Input: part model. Units: mm. Frame: model coordinates. A direction names the side the tool comes from. Coordinates: 2 decimals unless noted, no trailing zeros. Loops run counter-clockwise (first coordinate to the right, second up) from the corner with the lowest first, then second, coordinate; pieces in that order, holes last. Notation, with made-up numbers: (52.5, 26) -> (108.5, 26) arc R24 cw to (108.5, 59) -> close; hole circle Ø8 at (3, 87.25). An arc over 180 degrees is marked (long way). Answer as a JSON object with one key per item and string values.
from build123d import *

# Parameters (mm, degrees)
CROQUIS1_R              = 5.05
CROQUIS1_R_2            = 1.7500000000000002
SALIENTE_EXTRUIR1_DEPTH = 1.5
CROQUIS8_R              = 7
CROQUIS8_R_2            = 3.5499999999999994
SALIENTE_EXTRUIR5_DEPTH = 1.5
CROQUIS9_R              = 3
CORTAR_EXTRUIR3_DEPTH   = 1.5
CROQUIS10_R             = 3.55
SALIENTE_EXTRUIR6_DEPTH = 0.4
CHAFL_N1_SIZE           = 0.5


with BuildPart() as part:
    # Croquis1 → Saliente-Extruir1 (new body)
    with BuildSketch(Plane.XY):
        with BuildLine():
            Line((3.75, -2.0000000000000004), (19.8, -2))
            Line((19.8, -2), (19.8, 2))
            Line((19.8, 2), (8.90555127546391, 2))
            ThreePointArc((8.905551275463925, 1.9999999999999556), (6.887272990754048, 14.817665616090519), (-0.5849400470518447, 4.209554031171866))
            ThreePointArc((-0.5849400470518499, 4.209554031171828), (-3.484830188538549, -2.4327882269220193), (3.7499999999999996, -2.0000000000000013))
        make_face()
        with Locations((5.299999999999999, 8)):
            Circle(CROQUIS1_R, mode=Mode.SUBTRACT)
        Circle(CROQUIS1_R_2, mode=Mode.SUBTRACT)
    extrude(amount=SALIENTE_EXTRUIR1_DEPTH)

    # Croquis8 → Saliente-Extruir5 (add)
    with BuildSketch(Plane.XY.offset(1.5)):
        with Locations(Location((5.299999999999999, 8, 0), (0, 0, 212.785282787))):
            Circle(CROQUIS8_R)
        with Locations((5.299999999999999, 8)):
            Circle(CROQUIS8_R_2, mode=Mode.SUBTRACT)
    extrude(amount=SALIENTE_EXTRUIR5_DEPTH)

    # Croquis9 → Cortar-Extruir3 (cut)
    with BuildSketch(Plane.XY.offset(1.5)):
        Circle(CROQUIS9_R)
    extrude(amount=CORTAR_EXTRUIR3_DEPTH, mode=Mode.SUBTRACT)

    # Croquis10 → Saliente-Extruir6 (add)
    with BuildSketch(Plane(origin=(0, 0, 1.5), x_dir=(-1, 0, 0), z_dir=(0, 0, -1))):
        with Locations((-5.299999999999999, 8)):
            Circle(CROQUIS10_R)
    extrude(amount=-SALIENTE_EXTRUIR6_DEPTH)

    # Simetría1: part across plane


with BuildPart() as part_1:
    add(part.part)
    add(part.part.mirror(Plane(origin=(19.8, 0, 1.5), x_dir=(0, 0, 1), z_dir=(1, 0, 0))))

    # Chaflán1
    chafl_n1_edges = [part_1.edges().sort_by_distance(p)[0] for p in [
        (19.8, -2.000000000000001, 0),
        (-3.484830188538548, -2.4327882269220202, 0),
        (6.887272990754054, 14.817665616090517, 0),
        (41.35, 2.1e-16, 0),
        (39.35, 8, 0),
        (32.712727009245945, 14.817665616090517, 0),
        (43.08483018853855, -2.4327882269220202, 0),
        (0.2499999999999991, 8, 0),
        (-1.7500000000000002, 2.1e-16, 0),
        (19.8, 1.999999999999977, 0),
    ]]
    chamfer(chafl_n1_edges, length=CHAFL_N1_SIZE)


solid = part_1.part
1. Access query for faces 1 (the face through (4.6, 13, 1)), 2 (the face through (9, 8, 3)), 3 (the face through (20, 2, 1)), 4 (the face through (31.02, 6.64, 2.44)). Directions: +Z, -Z, +X, -X, +Y, -Y. A direction counts if a zero-diameter tool reaches every point of the face in a straight line with its end or side. Return the directions, or none.
Reply:
{"face 1": "-Z", "face 2": "+Z, +X, -X, +Y, -Y", "face 3": "+Z, -Z", "face 4": "+Z"}
2. Pin query (flat end, axial travel): P1, Ø5.5, axis at x = 39.6, y = 0, coming from the +Z side; P2, Ø0.8, axis at x = 15, z = 1, coming from the +Y side; P3, Ø0.8, axis at x = 13, z = 1, coming from the -Y side. Return the tip coordinate at first contact, or that it passes through.
Reply:
{"P1": "stops at z = 1.5", "P2": "stops at y = 2", "P3": "stops at y = -2"}
3. Section query B-B (x = 13.5). Return loops of the section in (y, z).
Reply:
{"outline": "(-2, 0.5) -> (-1.5, 0) -> (1.5, 0) -> (2, 0.5) -> (2, 1.5) -> (-2, 1.5) -> close"}
4. Mould query, pull axis Y, two halves, no side actions, for faces 5 (the face through (37.93, 2.49, 2.24)), 6 (the face through (31, 6, 3)), 7 (the face through (5, 8, 1.5)), 8 (the face through (31.322, 13.937, 0.142)). Classes: pulls with the +Y half, pulls with the -Y half, needs draft (parallel to the pull), parting line crosses it, or undercut.
Reply:
{"face 5": "pulls with the -Y half", "face 6": "needs draft", "face 7": "undercut", "face 8": "undercut"}
5. Line query: line 1 along Y through (x, z) = (5.3, 2.4); line 2 along X through (y, z) = (-0.5, 1.45); line 3 along Y through (x, z) = (34.3, 1.1). Output: solid intervals per line, ascending.
Reply:
{"line 1": "y = 1 to 4.45, 11.55 to 15", "line 2": "x = -4.22 to -1.68, 1.68 to 37.92, 41.28 to 43.82", "line 3": "y = -2 to 2.95, 13.05 to 15"}
